Autodesk Inventor part; units mm, degrees
ref_plane "YZ Plane" through (0, 0, 0) normal (1, 0, 0) x (0, 1, 0)
ref_plane "XZ Plane" through (0, 0, 0) normal (0, 1, 0) x (-1, 0, 0)
ref_plane "XY Plane" through (0, 0, 0) normal (0, 0, 1) x (1, 0, 0)
sketch "Skizze2" plane through (0, 0, 0) normal (0, 1, 0) x (-1, 0, 0)
  line L0 (-1.5875, -2.3813) -> (-1.5875, 2.3812)
  line L1 (-1.5875, 2.3812) -> (-3.5719, 2.3812)
  arc A0 (-3.5719, 2.3812) -> (-4.3656, 1.5875) centre (-3.5719, 1.5875) ccw
  line L2 (-4.3656, 1.5875) -> (-4.3656, 0.7937)
  line L3 (-4.3656, 0.7937) -> (-3.175, 0.7937)
  line L4 (-3.175, 0.7937) -> (-3.175, -0.7937)
  line L5 (-3.175, -0.7937) -> (-4.3656, -0.7937)
  line L6 (-4.3656, -0.7937) -> (-4.3656, -1.5875)
  line L7 (-1.5875, -2.3813) -> (-3.5719, -2.3813)
  arc A1 (-4.3656, -1.5875) -> (-3.5719, -2.3813) centre (-3.5719, -1.5875) ccw
  line L8 (0, 2.3813) -> (0, -2.3813)
  line L9 (-5.436, 0) -> (0.906, 0)
  point P0 (0, 0)
  point P1 (0, 0)
  dimension "d0" = 3.175
  dimension "d1" = 6.35
  dimension "d2" = 8.7312
  dimension "d3" = 1.5875
  dimension "d4" = 4.7625
  dimension "d5" = 0.7937
revolve "Umdrehung1" add sketch "Skizze2" angle 360 about axis through (0, 0, 2.3813) along (0, 0, -1)
properties part number "Gummitülle 3mm" material "Gummi"
CAD build for the part. Positions are in the model's coordinates, mm. A direction names the side the tool comes from. Round coordinates to 2 decimals unless told otherwise and drop trailing zeros. Loops run counter-clockwise (first coordinate to the right, second up) from the corner with the lowest first, then second, coordinate; pieces in that order, holes last. Notation, with made-up numbers: M 51.25,1 L 62.25,1 A16 ccw 62.25,12 Z; hole C 54.5,-38 d3. An arc over 180 degrees is marked long. One line per question, with ' | ' between items. Start each with the question number.
Item 1: Cut at A-A, the plane y = 0. Write the cut outline in (x, z) (1 decimal), plus the area to 3 significant figures.
Item 2: Two-plate mould, pull along Z, no slides. Class faces 1 (the cylindrical face through (-0.57, -4.33, -1.2)), 2 (the flat face through (2, 3, 0.794)), 3 (the cylindrical face through (-0.69, 3.1, -0.01)), 4 (the flat face through (2, 1, 2.381)): pulls with the +Z half, pulls with the -Z half, needs draft (parallel to the pull), parting line crosses it, or undercut.
Item 3: Cut at C-C, the plane z = 1.35. Write the cut outline in (x, y) (1 decimal), plus the area to 3 significant figures.
Item 4: Wall check: line 1 (Y direction, x = 0, z = -1.3); line 2 (Z direction, x = 1, y = -3.25). Give the ranges that are in metal, low to high.
Item 5: Which spindle directions (+Z, -Z, +X, -X, +Y, -Y) get a long thin tool onto all of the face, cutting with end or side? Do faces 5 (the flat face through (2, 3, -0.794)), 6 (the flat face through (2, 1, -2.381)). Say none if no direction does.
Item 6: Pin check, flat tips, straight feed: pin 1 Ø1 at (y, z) = (-0.5, -2) entering from +X; pin 2 Ø1 at (y, z) = (-1, 0.5) entering from -X. Stop position of each tip, or through.
Responses:
1) outline: M -4.4,-1.6 A0.8 ccw -3.6,-2.4 L -1.6,-2.4 L -1.6,2.4 L -3.6,2.4 A0.8 ccw -4.4,1.6 L -4.4,0.8 L -3.2,0.8 L -3.2,-0.8 L -4.4,-0.8 Z; M 1.6,-2.4 L 3.6,-2.4 A0.8 ccw 4.4,-1.6 L 4.4,-0.8 L 3.2,-0.8 L 3.2,0.8 L 4.4,0.8 L 4.4,1.6 A0.8 ccw 3.6,2.4 L 1.6,2.4 Z | area: 22.1 mm²
2) face 1: needs draft | face 2: undercut | face 3: undercut | face 4: pulls with the +Z half
3) outline: C 0,0 d8.7; hole C 0,0 d3.2 | area: 52.0 mm²
4) line 1: y = -4.37 to -1.59, 1.59 to 4.37 | line 2: z = -2.38 to -0.79, 0.79 to 2.38
5) face 5: none | face 6: -Z, +X, -X, +Y, -Y
6) pin 1: stops at x = 4.36 | pin 2: stops at x = -4.32
